Can you work these out from the model? Positions are in its coordinate system, mm. Face numbers are marked on the shaded views. A direction names the side the tool comes from. Coordinates: 2 decimals unless noted, no trailing zeros. Write each loop counter-clockwise with the first axis right and the second up, starting at its lowest first coordinate (ties: lowest second). Pieces come first, ordered by that corner, then holes. Notation, with made-up numbers: (27, 30) - (53, 30) arc R27 ccw to (53, 58) - close; hole circle Ø2 at (67.5, 84.25). An arc over 180 degrees is marked (long way). One line per question, with ' | ' between items. Start each with the question number.
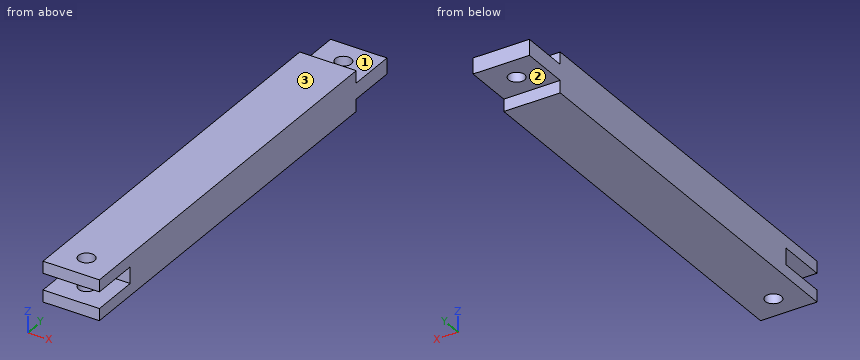
Autodesk Inventor part; units mm, degrees
ref_plane "YZ Plane" through (0, 0, 0) normal (1, 0, 0) x (0, 1, 0)
ref_plane "XZ Plane" through (0, 0, 0) normal (0, 1, 0) x (-1, 0, 0)
ref_plane "XY Plane" through (0, 0, 0) normal (0, 0, 1) x (1, 0, 0)
sketch "Sketch1" plane through (0, 0, 0) normal (0, 1, 0) x (-1, 0, 0)
  line L0 (-3.5, 2.5) -> (3.5, 2.5)
  line L1 (3.5, 2.5) -> (3.5, -2.5)
  line L2 (3.5, -2.5) -> (-3.5, -2.5)
  line L3 (-3.5, -2.5) -> (-3.5, 2.5)
  line L4 (-3.5, 2.5) -> (3.5, -2.5) construction
  line L5 (3.5, 2.5) -> (-3.5, -2.5) construction
  point P0 (0, 0)
  dimension "d0" = 5
  dimension "d1" = 7
extrude "Extrusion1" add sketch "Sketch1" along normal blind 50
sketch "Sketch2" plane through (0, 50, 0) normal (0, 1, 0) x (1, 0, 0)
  line L0 (-3.5, -2.5) -> (3.5, -2.5)
  line L1 (3.5, -2.5) -> (3.5, 2.5)
  line L2 (3.5, 2.5) -> (-3.5, 2.5)
  line L3 (-3.5, -2.5) -> (3.5, -2.5)
  line L4 (3.5, -2.5) -> (3.5, -0.98)
  line L5 (3.5, -0.98) -> (-3.5, -0.98)
  line L6 (-3.5, -0.98) -> (-3.5, -2.5)
  line L7 (-3.5, 2.5) -> (3.5, 2.5)
  line L8 (3.5, 2.5) -> (3.5, 0.98)
  line L9 (3.5, 0.98) -> (-3.5, 0.98)
  line L10 (-3.5, 0.98) -> (-3.5, 2.5)
  point P0 (0, 0)
  dimension "d4" = 1.52
  dimension "d5" = 1.52
extrude "Extrusion2" cut sketch "Sketch2" against normal blind 6
sketch "Sketch3" plane through (-3.5, 50, 0.98) normal (0, 0, 1) x (1, 0, 0)
  line L0 (0, 0) -> (7, 0)
  line L1 (7, 0) -> (7, -6)
  circle A0 centre (3.5, -3) radius 1
  point P0 (3.5, -50)
  dimension "d8" = 2
  dimension "d9" = 3.5
  dimension "d10" = 3
extrude "Extrusion3" cut sketch "Sketch3" against normal through all
sketch "Sketch4" plane through (0, 0, 0) normal (0, -1, 0) x (1, 0, 0)
  line L0 (3.5, 2.5) -> (-3.5, 2.5)
  line L1 (-3.5, 2.5) -> (-3.5, -2.5)
  line L2 (-3.5, -2.5) -> (3.5, -2.5)
  line L3 (3.5, 0.98) -> (3.5, -0.98)
  line L4 (-3.5, 2.5) -> (3.5, 2.5)
  line L5 (3.5, 2.5) -> (3.5, 1.02)
  line L6 (3.5, 1.02) -> (-3.5, 1.02)
  line L7 (-3.5, 1.02) -> (-3.5, 2.5)
  line L8 (-3.5, -2.5) -> (3.5, -2.5)
  line L9 (3.5, -2.5) -> (-3.5, -2.5)
  line L10 (-3.5, -2.5) -> (-3.5, -1.02)
  line L11 (-3.5, -1.02) -> (3.5, -1.02)
  line L12 (3.5, -1.02) -> (3.5, -2.5)
  point P0 (0, 0)
  dimension "d13" = 1.48
  dimension "d14" = 1.48
extrude "Extrusion4" add sketch "Sketch4" along normal blind 6
sketch "Sketch5" plane through (-3.5, 0, 1.02) normal (0, 0, -1) x (1, 0, 0)
  line L0 (7, 0) -> (0, 0)
  line L1 (7, 0) -> (7, 6)
  circle A0 centre (3.5, 3) radius 1
  point P0 (3.5, 0)
  dimension "d17" = 3
  dimension "d18" = 3.5
  dimension "d19" = 2
extrude "Extrusion6" cut sketch "Sketch5" along normal through all both and the other way through all
properties part number "LD_holder_p4"
(1) If we section it at B-B on y = 47: List the corners of the cut face in (x, z) for me.
(2) If we section it at A-A on y = -3: List the corners of the cut face in (x, z) for me.
(3) If we section it at D-D on z = 0.1: List the corners of the cut face in (x, y) for me, plus the area to 3 significant figures.
(4) If I drill on probe 1 along Z at (x, y) = (-0.5, -1.5); probe 2 along Y at (x, z) = (0, 0.15); probe 3 along Y at (x, z) = (0, 1.45), over which ranges is the centre line in solid material (lowest first)?
(5) Which directions (+Z, -Z, +X, -X, +Y, -Y) give clear straight access to the entire face, cutting with the end or side of a thin tool? Please do the marked faces 1, 2 and 3.
(6) If we section it at C-C on x = 0: List the corners of the cut face in (y, z) for me, plus the area to 3 significant figures.
(7) I'm going to push flat-ended pins straight in: pin 1 (3 mm diameter, centred on x = 1.5, y = 46.5, fed in from +Z); pin 2 (3 mm diameter, centred on x = -1, y = 48, fed in from -Z); pin 3 (0.8 mm diameter, centred on x = -1, z = -1.5, fed in from +Y). Where does each tip first touch, or does it pass through?
Values:
1) outline: (-3.5, -0.98) - (-1, -0.98) - (-1, 0.98) - (-3.5, 0.98) - close; (1, -0.98) - (3.5, -0.98) - (3.5, 0.98) - (1, 0.98) - close
2) outline: (-3.5, -2.5) - (-1, -2.5) - (-1, -1.02) - (-3.5, -1.02) - close; (-3.5, 1.02) - (-1, 1.02) - (-1, 2.5) - (-3.5, 2.5) - close; (1, -2.5) - (3.5, -2.5) - (3.5, -1.02) - (1, -1.02) - close; (1, 1.02) - (3.5, 1.02) - (3.5, 2.5) - (1, 2.5) - close
3) outline: (-3.5, 0) - (3.5, 0) - (3.5, 50) - (-3.5, 50) - close; hole circle Ø2 at (0, 47) | area: 347 mm2
4) probe 1: -2.5 to -1.02, 1.02 to 2.5 | probe 2: 0 to 46, 48 to 50 | probe 3: -6 to -4, -2 to 44
5) face 1: +Z, +X, -X, +Y | face 2: -Z, +X, -X, +Y | face 3: +Z, +X, -X, +Y, -Y
6) outline: (-6, -2.5) - (-4, -2.5) - (-4, -1.02) - (-6, -1.02) - close; (-6, 1.02) - (-4, 1.02) - (-4, 2.5) - (-6, 2.5) - close; (-2, -2.5) - (44, -2.5) - (44, -0.98) - (46, -0.98) - (46, 0.98) - (44, 0.98) - (44, 2.5) - (-2, 2.5) - (-2, 1.02) - (0, 1.02) - (0, -1.02) - (-2, -1.02) - close; (48, -0.98) - (50, -0.98) - (50, 0.98) - (48, 0.98) - close | area: 240 mm2
7) pin 1: z = 0.98 | pin 2: z = -0.98 | pin 3: y = 44
